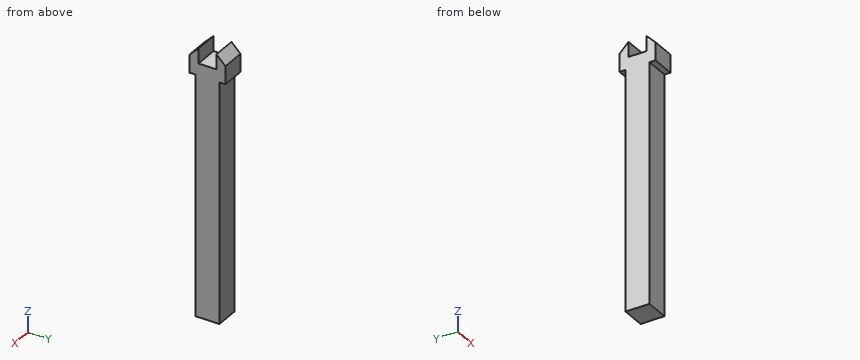
from build123d import *

# Parameters (mm, degrees)
SKETCH1_W           = 20
SKETCH1_H           = 20
BOSS_EXTRUDE1_DEPTH = 200
SKETCH2_W           = 20
SKETCH2_H           = 30
BOSS_EXTRUDE2_DEPTH = 25
SKETCH3_W           = 20
SKETCH3_H           = 15
CUT_EXTRUDE1_DEPTH  = 15
CHAMFER1_SIZE       = 10
CHAMFER3_SIZE       = 10


with BuildPart() as part:
    # Sketch1 → Boss-Extrude1 (new body)
    with BuildSketch(Plane.XY):
        Rectangle(SKETCH1_W, SKETCH1_H)
    extrude(amount=BOSS_EXTRUDE1_DEPTH)

    # Sketch2 → Boss-Extrude2 (add)
    with BuildSketch(Plane.XY.offset(200)):
        Rectangle(SKETCH2_W, SKETCH2_H)
    extrude(amount=BOSS_EXTRUDE2_DEPTH)

    # Sketch3 → Cut-Extrude1 (cut)
    with BuildSketch(Plane.XY.offset(225)):
        Rectangle(SKETCH3_W, SKETCH3_H)
    extrude(amount=-CUT_EXTRUDE1_DEPTH, mode=Mode.SUBTRACT)

    # Chamfer1
    # the kernel refuses this chamfer: 10 mm, written as the material it takes off along each edge
    with BuildSketch(Plane(origin=(35.71682988, 15, 225), x_dir=(0, -0.9996219169112968, 0.0274958766105877), z_dir=(-1, 0, 0))) as chamfer1_piece_1:
        Polygon((CHAMFER1_SIZE * 0.999621916911, -CHAMFER1_SIZE * 0.0274958766106), (-CHAMFER1_SIZE * 0.0274958766106, -CHAMFER1_SIZE * 0.999621916911), (0, 0), align=None)
    extrude(amount=71.433659759, mode=Mode.SUBTRACT)

    # Chamfer3
    # the kernel refuses this chamfer: 10 mm, written as the material it takes off along each edge
    with BuildSketch(Plane(origin=(-35.71682988, -15, 225), x_dir=(0, -0.027495876610586282, -0.9996219169112968), z_dir=(1, 0, 0))) as chamfer3_piece_1:
        Polygon((CHAMFER3_SIZE * 0.999621916911, CHAMFER3_SIZE * 0.0274958766106), (-CHAMFER3_SIZE * 0.0274958766106, CHAMFER3_SIZE * 0.999621916911), (0, 0), align=None)
    extrude(amount=71.433659759, mode=Mode.SUBTRACT)


solid = part.part
Build history of the part. All positions in model axes, mm. Give positions to 0.01 mm unless a question says otherwise; leave off trailing zeros. Write each loop counter-clockwise with the first axis right and the second up, starting at its lowest first coordinate (ties: lowest second). Pieces come first, ordered by that corner, then holes. Notation, with made-up numbers: (-20.75, -25.75) - (1.25, -25.75) arc R30 cw to (1.25, -3.75) - close; hole circle Ø7 at (-6.5, 20.25). An arc over 180 degrees is marked (long way). Use one line per item in the form item = value. Start each with the question number.
1. Drop flat-ended pins along their axis: pin 1 Ø6 at (x, z) = (1.5, 59) entering from +Y; pin 2 Ø10 at (x, z) = (4, 69.5) entering from -Y; pin 3 Ø4 at (x, y) = (-1, 13.5) entering from -Z. Give the stop position or say it passes through.
2. Probe line 1 (Y direction, x = -9, z = 163); line 2 (Z direction, x = 6, y = 6); line 3 (Z direction, x = -7.5, y = -9). List the from-to ranges inside material, lowest first. Write a range as [from, to].
3. Band-saw the part on C-C on z = 173.5. Write the cut outline in (x, y).
4. Band-saw the part on B-B on y = 4. Write the cut outline in (x, z), plus the area to 3 significant figures.
5. Band-saw the part on A-A on x = 3.75. Write the cut outline in (y, z).
Conclusion:
q1.pin_1 = 10
q1.pin_2 = -10
q1.pin_3 = 200
q2.line_1 = [-10, 10]
q2.line_2 = [0, 210]
q2.line_3 = [0, 221]
q3.outline = (-10, -10) - (10, -10) - (10, 10) - (-10, 10) - close
q4.outline = (-10, 0) - (10, 0) - (10, 210) - (-10, 210) - close
q4.area = 4,200 mm²
q5.outline = (-15, 200) - (-10, 200) - (-10, 0) - (10, 0) - (10, 200) - (15, 200) - (15, 215) - (7.5, 222.5) - (7.5, 210) - (-7.5, 210) - (-7.5, 222.5) - (-15, 215) - close
